Read the model definition and answer for the solid it produces. Units are mm, in the model's axes. A direction names the side the tool comes from. Coordinates: 2 decimals unless noted, no trailing zeros. Order: outer loops, then holes, each group sorted by start corner. A loop starts at its lowest first (then second) coordinate and runs counter-clockwise, first axis right, second up.
```python
from build123d import *

# Parameters (mm, degrees)
BOSS_EXTRUDE1_DEPTH = 50.8
SKETCH3_R           = 2.500488375
SKETCH3_R_2         = 1.357488375
SKETCH3_R_3         = 2.499609862
SKETCH3_R_4         = 2.52658695
SKETCH3_R_5         = 2.538600877
BOSS_EXTRUDE2_DEPTH = 3.175
BOSS_EXTRUDE3_START = 3.175
SKETCH3_3_R         = 1.357488375
SKETCH3_3_R_2       = 1.356609862
SKETCH3_3_R_3       = 1.38358695
SKETCH3_3_R_4       = 1.395600877
BOSS_EXTRUDE3_DEPTH = 2.54
SKETCH4_R           = 2.5
CUT_EXTRUDE1_DEPTH  = 10


with BuildPart() as part:
    # Sketch1 → Boss-Extrude1 (new body)
    with BuildSketch(Plane.XY):
        Polygon((12.7, 70.0786), (12.7, 54.2036), (7.3025, 54.2036), (7.3025, 52.5018), (12.7, 52.5018), (12.7, 36.6268), (7.3025, 36.6268), (7.3025, 34.925), (12.7, 34.925), (12.7, 0), (0, 0), (0, 73.2536), (66.167, 73.2536), (66.167, 0), (53.467, 0), (53.467, 34.925), (58.8645, 34.925), (58.8645, 36.6268), (53.467, 36.6268), (53.467, 52.5018), (58.8645, 52.5018), (58.8645, 54.2036), (53.467, 54.2036), (53.467, 70.0786), align=None)
    extrude(amount=BOSS_EXTRUDE1_DEPTH)

    # Sketch3 → Boss-Extrude2 (add)
    with BuildSketch(Plane(origin=(0, 73.2536, 0), x_dir=(1, 0, 0), z_dir=(0, 1, 0))):
        with Locations(Location((16.012534946, -8.068344252, 0), (0, 0, 90))):
            Circle(SKETCH3_R)
        with Locations((16.012534946, -8.068344252)):
            Circle(SKETCH3_R_2, mode=Mode.SUBTRACT)
        with Locations((16.012534946, -8.068344252)):
            Circle(SKETCH3_R_2)
        with Locations(Location((15.66334422, -42.22825299, 0), (0, 0, 90))):
            Circle(SKETCH3_R_3)
        with Locations(Location((50.174167917, -42.233596828, 0), (0, 0, 90))):
            Circle(SKETCH3_R_4)
        with Locations(Location((49.881189528, -8.139195897, 0), (0, 0, 90))):
            Circle(SKETCH3_R_5)
    extrude(amount=BOSS_EXTRUDE2_DEPTH)

    # Sketch3<3> → Boss-Extrude3 (add)
    with BuildSketch(Plane(origin=(0, 73.2536, 0), x_dir=(1, 0, 0), z_dir=(0, 1, 0)).offset(BOSS_EXTRUDE3_START)):
        with Locations(Location((16.012534946, -8.068344252, 0), (0, 0, 270))):
            Circle(SKETCH3_3_R)
        with Locations(Location((15.66334422, -42.22825299, 0), (0, 0, 270))):
            Circle(SKETCH3_3_R_2)
        with Locations(Location((50.174167917, -42.233596828, 0), (0, 0, 270))):
            Circle(SKETCH3_3_R_3)
        with Locations(Location((49.881189528, -8.139195897, 0), (0, 0, 270))):
            Circle(SKETCH3_3_R_4)
    extrude(amount=BOSS_EXTRUDE3_DEPTH)

    # Sketch4 → Cut-Extrude1 (cut)
    with BuildSketch(Plane.XZ):
        with Locations(Location((6.35, 38.1, 0), (0, 0, 270))):
            Circle(SKETCH4_R)
        with Locations(Location((6.35, 12.7, 0), (0, 0, 270))):
            Circle(SKETCH4_R)
        with Locations(Location((59.817, 38.1, 0), (0, 0, 270))):
            Circle(SKETCH4_R)
        with Locations(Location((59.817, 12.7, 0), (0, 0, 270))):
            Circle(SKETCH4_R)
    extrude(amount=-CUT_EXTRUDE1_DEPTH, mode=Mode.SUBTRACT)


solid = part.part
```
1) Straight lines are drawn through the part: line 1 (X direction, y = 5, z = 12.7); line 2 (Y direction, x = 8.5, z = 6) (3 decimals); line 3 (X direction, y = 42.5, z = 46.5). For each, find the intervals that lie inside material, in ascending order.
A:
line 1: x = 0 to 3.85, 8.85 to 12.7, 53.47 to 57.32, 62.32 to 66.17
line 2: y = 0 to 34.925, 36.627 to 52.502, 54.204 to 73.254
line 3: x = 0 to 12.7, 53.47 to 66.17
2) Determine the mould class of faces 5 (the flat face through (6, 10, 38)), 6 (the flat face through (12.7, 45, 25)), 7 (the flat face through (10, 34.925, 25)) for opening direction Y: pulls with the +Y half, pulls with the -Y half, needs draft (parallel to the pull), parting line crosses it, or undercut.
A:
face 5: pulls with the -Y half
face 6: needs draft
face 7: undercut
3) A cutting plane is placed at A-A, the plane y = 48. Determine the outline of the cut face in (x, z), and give its area (3 significant figures).
A:
outline: (0, 0) - (12.7, 0) - (12.7, 50.8) - (0, 50.8) - close; (53.47, 0) - (66.17, 0) - (66.17, 50.8) - (53.47, 50.8) - close
area: 1,290 mm2
4) Flat-ended cylindrical pins translate along their axes: pin 1 Ø8 at (x, z) = (51.5, 36) entering from +Y; pin 2 Ø0.5 at (y, z) = (35.5, 33.5) entering from -X; pin 3 Ø10 at (x, z) = (28, 45.5) entering from -Y; pin 4 Ø2.5 at (x, z) = (59.5, 12) entering from -Y. Find the tip coordinate at first contact, or state that the pin passes through.
A:
pin 1: stops at y = 76.43
pin 2: stops at x = 0
pin 3: stops at y = 70.08
pin 4: stops at y = 10
5) A cutting plane is placed at B-B, the plane z = 21. Determine the outline of the cut face in (x, y) (1 decimal).
A:
outline: (0, 0) - (12.7, 0) - (12.7, 34.9) - (7.3, 34.9) - (7.3, 36.6) - (12.7, 36.6) - (12.7, 52.5) - (7.3, 52.5) - (7.3, 54.2) - (12.7, 54.2) - (12.7, 70.1) - (53.5, 70.1) - (53.5, 54.2) - (58.9, 54.2) - (58.9, 52.5) - (53.5, 52.5) - (53.5, 36.6) - (58.9, 36.6) - (58.9, 34.9) - (53.5, 34.9) - (53.5, 0) - (66.2, 0) - (66.2, 73.3) - (0, 73.3) - close
6) Which of the six approach directions +Z, -Z, +X, -X, +Y, -Y give full straight-line access (tool end or side, diameter ignored) to faces 1 (the flat face through (12.7, 62, 25)), 2 (the cylindrical face through (7.101, 4.93, 35.715)), 3 (the flat face through (10, 54.204, 25)), 4 (the cylindrical face through (50.824, 77.681, 7.111))?
A:
face 1: +Z, -Z, -Y
face 2: -Y
face 3: +Z, -Z
face 4: +Y
7) A cutting plane is placed at C-C, the plane x = 6.35. Determine the outline of the cut face in (y, z).
A:
outline: (0, 0) - (73.25, 0) - (73.25, 50.8) - (0, 50.8) - (0, 40.6) - (10, 40.6) - (10, 35.6) - (0, 35.6) - (0, 15.2) - (10, 15.2) - (10, 10.2) - (0, 10.2) - close
